Geometry: final body of the model. Coordinates: model frame, mm. A direction names the side the tool comes from. Give positions to 0.01 mm unless a question says otherwise; leave off trailing zeros. Write each loop counter-clockwise with the first axis right and the second up, starting at its lowest first coordinate (ties: lowest second). Pieces come first, ordered by that corner, then holes.
Q1. Cut plane D-D on y = 25. Return the cut outline in (x, z), plus the area to 3 significant figures.
Q2. Cut plane C-C on x = 16.5. Return the cut outline in (y, z).
Q3. Line query: L1, parallel to X at y = 22.5, z = 35; L2, parallel to X at y = 4, z = 5; L3, parallel to Y at x = 12.5, z = 11.5. Output: solid intervals per line, ascending.
Q4. Reachability of faces 1 (the face through (24, 0, 20)), 2 (the face through (20, 20, 30)) from +Z, -Z, +X, -X, +Y, -Y: full face, straight path, thin tool, end or side. Return the list, or none.
Q5. Cut plane B-B on z = 4. Return the cut outline in (x, y), plus the area to 3 significant figures.
Q6. Cut plane A-A on y = 30. Return the cut outline in (x, z).
Q7. Pin query (flat end, axial travel): pin 1 (16 mm diameter, centred on x = 5.5, y = 22.5, fed in from +Z); pin 2 (4 mm diameter, centred on y = 6.5, z = 36, fed in from -X). Return the tip coordinate at first contact, or that it passes through.
```python
from build123d import *

# Parameters (mm, degrees)
SKETCH1_W           = 40
SKETCH1_H           = 40
BOSS_EXTRUDE1_DEPTH = 40
CUT_EXTRUDE1_DEPTH  = 40
SKETCH3_W           = 20
SKETCH3_H           = 20
CUT_EXTRUDE2_DEPTH  = 40
CUT_EXTRUDE3_DEPTH  = 40


with BuildPart() as part:
    # Sketch1 → Boss-Extrude1 (new body)
    with BuildSketch(Plane.XY):
        with Locations((20, 20)):
            Rectangle(SKETCH1_W, SKETCH1_H)
    extrude(amount=BOSS_EXTRUDE1_DEPTH)

    # Sketch2 → Cut-Extrude1 (cut)
    with BuildSketch(Plane.XY.offset(40)):
        Polygon((0, 0), (20, 40), (0, 40), align=None)
    extrude(amount=-CUT_EXTRUDE1_DEPTH, mode=Mode.SUBTRACT)

    # Sketch3 → Cut-Extrude2 (cut)
    with BuildSketch(Plane(origin=(0, 0, 0), x_dir=(-1, 0, 0), z_dir=(0, -1, 0))):
        with Locations((-10, -30)):
            Rectangle(SKETCH3_W, SKETCH3_H)
    extrude(amount=-CUT_EXTRUDE2_DEPTH, mode=Mode.SUBTRACT)

    # Sketch4 → Cut-Extrude3 (cut)
    with BuildSketch(Plane.XZ):
        Polygon((20, 0), (0, 20), (0, 0), align=None)
    extrude(amount=-CUT_EXTRUDE3_DEPTH, mode=Mode.SUBTRACT)


solid = part.part
```
Data:
1. outline: (12.5, 7.5) - (20, 0) - (40, 0) - (40, 40) - (20, 40) - (20, 20) - (12.5, 20) - close
1. area: 922 mm2
2. outline: (0, 3.5) - (33, 3.5) - (33, 20) - (0, 20) - close
3. L1: x = 20 to 40
3. L2: x = 15 to 40
3. L3: y = 0 to 25
4. face 1: +Z, -Z, +X, -X, -Y
4. face 2: +Z, -X, +Y, -Y
5. outline: (16, 0) - (40, 0) - (40, 40) - (20, 40) - (16, 32) - close
5. area: 944 mm2
6. outline: (15, 5) - (20, 0) - (40, 0) - (40, 40) - (20, 40) - (20, 20) - (15, 20) - close
7. pin 1: stops at z = 20
7. pin 2: stops at x = 20
